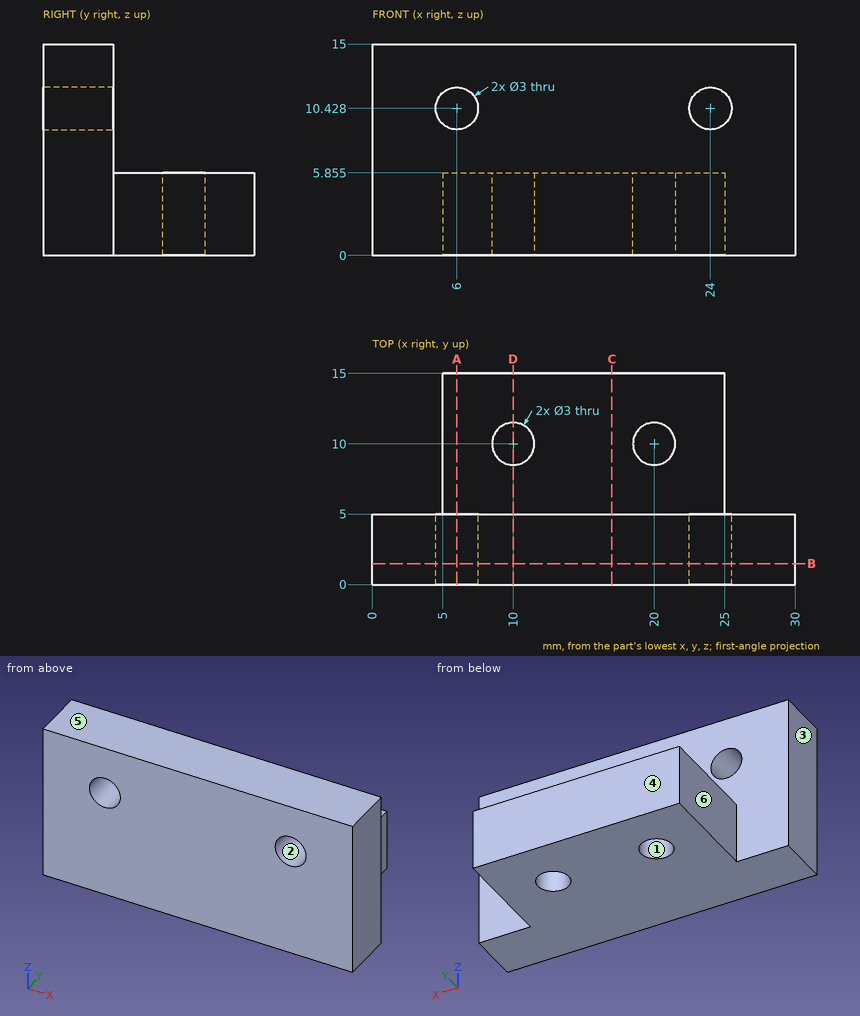
Source: three-view drawing plus pictorial views. Frame: mm from the lowest corner of the part. A direction names the side the tool comes from. Give positions to 0.01 mm unless a question says otherwise; leave off trailing zeros. Order: outer loops, then holes, each group sorted by start corner. A loop starts at its lowest first (then second) coordinate and runs counter-clockwise, first axis right, second up. Notation, with made-up numbers: (-16.5, -23) -> (30.5, -23) arc R20 cw to (30.5, 9) -> close; hole circle Ø3 at (68, 50). An arc over 180 degrees is marked (long way). Write each question's results on one line, items separated by ' | '. Start each with the question number.
Item 1: Mould query, pull axis X, two halves, no side actions, for the marked faces 1, 2, 3 and 4. Classes: pulls with the +X half, pulls with the -X half, needs draft (parallel to the pull), parting line crosses it, or undercut.
Item 2: Cut plane B-B on y = 1.5. Return the cut outline in (x, z), then the cut area to 3 significant figures.
Item 3: Cut plane A-A on x = 6. Return the cut outline in (y, z) (1 decimal).
Item 4: Contact query for flat-ended pins moving along their axis: P1, Ø4, axis at x = 20, y = 10, coming from the -Z side; P2, Ø2, axis at x = 23.5, z = 8.5, coming from the +Y side; P3, Ø1.8, axis at y = 8, z = 3, coming from the -X side; P4, Ø4, axis at x = 10, y = 10, coming from the +Z side (1 decimal). Output: stop coordinate, or through.
Item 5: Cut plane C-C on x = 17. Return the cut outline in (y, z) (1 decimal).
Item 6: Cut plane D-D on x = 10. Return the cut outline in (y, z) (1 decimal).
Item 7: Line query: line 1 (X direction, y = 1, z = 9.25); line 2 (Z direction, x = 18, y = 11.25) (1 decimal); line 3 (Y direction, x = 14, z = 9). Output: solid intervals per line, ascending.
Item 8: Set-up query: the marked faces 5 and 6. Return all of +Z, -Z, +X, -X, +Y, -Y with unobstructed straight access to the full face (end or side cutting, diameter ignored); none if empty.
Established:
1) face 1: undercut | face 2: undercut | face 3: pulls with the -X half | face 4: needs draft
2) outline: (0, 0) -> (30, 0) -> (30, 15) -> (0, 15) -> close; hole circle Ø3 at (6, 10.43); hole circle Ø3 at (24, 10.43) | area: 436 mm^2
3) outline: (0, 0) -> (15, 0) -> (15, 5.9) -> (5, 5.9) -> (5, 8.9) -> (0, 8.9) -> close; (0, 11.9) -> (5, 11.9) -> (5, 15) -> (0, 15) -> close
4) P1: z = 0 | P2: y = 5 | P3: x = 5 | P4: z = 5.9
5) outline: (0, 0) -> (15, 0) -> (15, 5.9) -> (5, 5.9) -> (5, 15) -> (0, 15) -> close
6) outline: (0, 0) -> (8.5, 0) -> (8.5, 5.9) -> (5, 5.9) -> (5, 15) -> (0, 15) -> close; (11.5, 0) -> (15, 0) -> (15, 5.9) -> (11.5, 5.9) -> close
7) line 1: 0 to 5.07, 6.93 to 23.07, 24.93 to 30 | line 2: 0 to 5.9 | line 3: 0 to 5
8) face 5: +Z, +X, -X, +Y, -Y | face 6: +Z, -Z, -X, +Y
